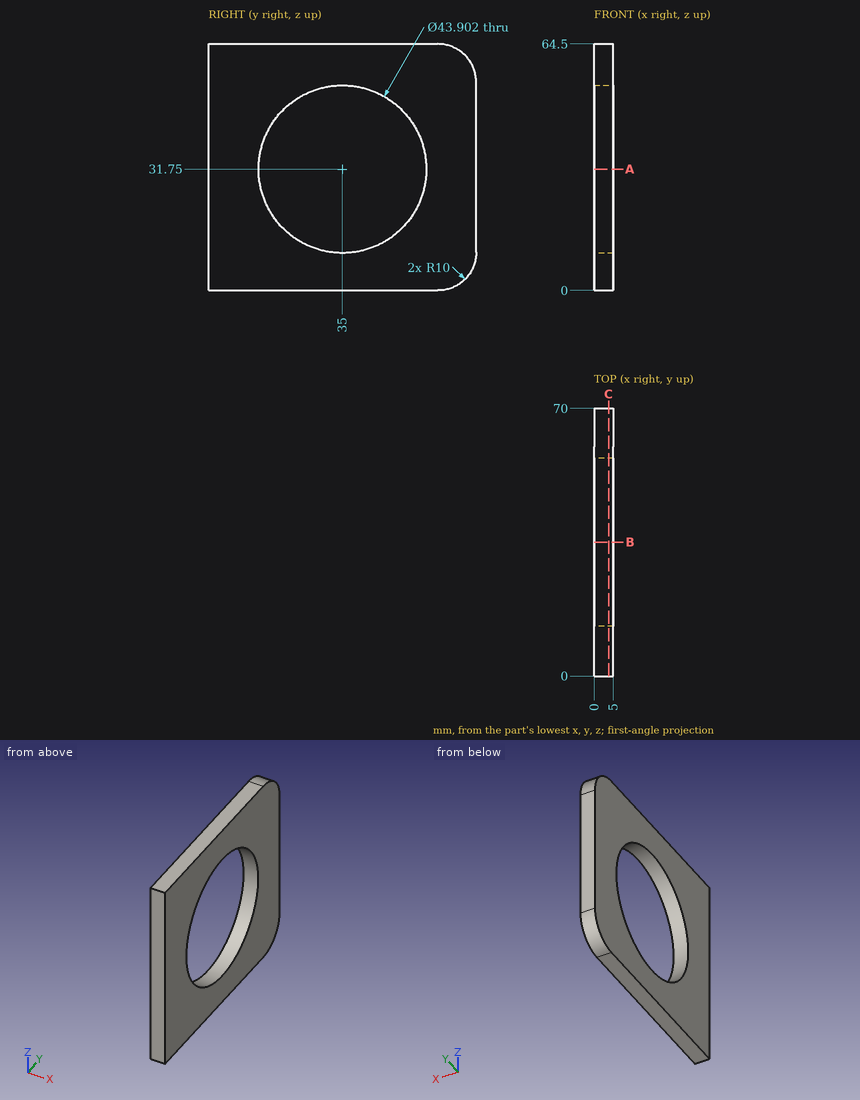
Check sheet for the drawn part. Datum: minimum x, y, z corner. Units: mm. Round coordinates to 2 decimals unless told otherwise and drop trailing zeros. Write each loop counter-clockwise with the first axis right and the second up, starting at its lowest first coordinate (ties: lowest second). Pieces come first, ordered by that corner, then holes. Notation, with made-up numbers: (43.25, 77.5) -> (75.25, 77.5) arc R18 ccw to (75.25, 88.5) -> close; hole circle Ø11 at (67.5, 51.25). An arc over 180 degrees is marked (long way). Write each question's results on one line, items separated by ' | '. Start each with the question number.
1. Cross-section at C-C (x = 3.8). Enter the section's corners in (y, z), then the cut area to 3 significant figures.
2. Material ranges on probe 1 along Y at (x, z) = (3.8, 31.75); probe 2 along Z at (x, y) = (2.25, 38) (3 decimals); probe 3 along Y at (x, z) = (3.15, 34) (1 decimal), recorded low to high. Write a range as from..to.
3. Cross-section at B-B (y = 35). Enter the section's corners in (x, z).
4. Cross-section at A-A (z = 31.75). Enter the section's corners in (x, y).
Solutions:
1) outline: (0, 0) -> (60, 0) arc R10 ccw to (70, 10) -> (70, 54.5) arc R10 ccw to (60, 64.5) -> (0, 64.5) -> close; hole circle Ø43.9 at (35, 31.75) | area: 2,960 mm2
2) probe 1: y = 0..13.05, 56.95..70 | probe 2: z = 0..10.005, 53.495..64.5 | probe 3: y = 0..13.2, 56.8..70
3) outline: (0, 0) -> (5, 0) -> (5, 9.8) -> (0, 9.8) -> close; (0, 53.7) -> (5, 53.7) -> (5, 64.5) -> (0, 64.5) -> close
4) outline: (0, 0) -> (5, 0) -> (5, 13.05) -> (0, 13.05) -> close; (0, 56.95) -> (5, 56.95) -> (5, 70) -> (0, 70) -> close
